For this review, take the finished solid that the model builds, in its own axes (mm). A direction names the side the tool comes from. Give positions to 0.01 mm unless a question says otherwise; leave off trailing zeros. Write each loop counter-clockwise with the first axis right and the second up, starting at its lowest first coordinate (ties: lowest second). Pieces come first, ordered by that corner, then holes.
1) We need section A-A on x = 13. Give the boundary of the cut face in (y, z), and give its area (3 significant figures).
2) Machinability: for faces 1 (the face through (24.53, 38.61, 4.93)), 2 (the face through (26.534, 92.543, 4.93)), which of the approach directions +Z, -Z, +X, -X, +Y, -Y give a long, thin tool a straight path to every point of the face, cutting with its end or side? Answer none if there is none.
3) We need section C-C on z = 5.5. Give the boundary of the cut face in (x, y).
4) We need section B-B on y = 65.5. Give the boundary of the cut face in (x, z).
5) Draft analysis for pull direction Y (two halves, no side actions). For faces 3 (the face through (26.525, 39.248, 4.93)), 4 (the face through (-49.662, 72.543, 4.93)), 5 (the face through (-52.564, 67, 5)), state which applies: pulls with the +Y half, pulls with the -Y half, needs draft (parallel to the pull), parting line crosses it, or undercut.
6) Wall thickness on line 1 along Y through (x, z) = (-12.5, 2); line 2 along X through (y, z) = (51, 7); line 3 along X through (y, z) = (73, 8.25): over which ranges is each line inside the solid? List them lowest first.
from build123d import *

# Parameters (mm, degrees)
RESSALTO_EXTRUS_O1_DEPTH = 10
CORTE_EXTRUS_O1_DEPTH    = 10


with BuildPart() as part:
    # Esboço1 → Ressalto-extrusão1 (new body)
    with BuildSketch(Plane.XY):
        with BuildLine():
            Line((-49.563885949, 93.398903013), (24.436114051, 93.398903013))
            ThreePointArc((24.436114051, 93.398903013), (26.557434395, 92.520223357), (27.436114051, 90.398903013))
            Line((27.436114051, 90.398903013), (27.436114051, 78.398903013))
            Line((27.436114051, 78.398903013), (27.436114051, 43.418903013))
            ThreePointArc((27.436114051, 43.418903013), (26.499191921, 39.192720396), (23.863990148, 35.758458582))
            Line((23.863990148, 35.758458582), (-48.991762046, 35.758458582))
            ThreePointArc((-48.991762046, 35.758458582), (-51.626963819, 39.192720396), (-52.563885949, 43.418903013))
            Line((-52.563885949, 43.418903013), (-52.563885949, 78.398903013))
            Line((-52.563885949, 78.398903013), (-52.563885949, 90.398903013))
            ThreePointArc((-52.563885949, 90.398903013), (-51.685206293, 92.520223357), (-49.563885949, 93.398903013))
        make_face()
    extrude(amount=RESSALTO_EXTRUS_O1_DEPTH)

    # Esboço2 → Corte-extrusão1 (cut)
    with BuildSketch(Plane(origin=(0, 0, 0), x_dir=(-1, 0, 0), z_dir=(0, 0, -1))):
        with BuildLine():
            Line((-22.436114051, 73.398903013), (47.563885949, 73.398903013))
            ThreePointArc((47.563885949, 73.398903013), (49.685206293, 72.520223357), (50.563885949, 70.398903013))
            Line((50.563885949, 70.398903013), (50.563885949, 40.758458582))
            ThreePointArc((50.563885949, 40.758458582), (49.685206293, 38.637138238), (47.563885949, 37.758458582))
            Line((47.563885949, 37.758458582), (-22.436114051, 37.758458582))
            ThreePointArc((-22.436114051, 37.758458582), (-24.557434395, 38.637138238), (-25.436114051, 40.758458582))
            Line((-25.436114051, 40.758458582), (-25.436114051, 70.398903013))
            ThreePointArc((-25.436114051, 70.398903013), (-24.557434395, 72.520223357), (-22.436114051, 73.398903013))
        make_face()
    extrude(amount=-CORTE_EXTRUS_O1_DEPTH, mode=Mode.SUBTRACT)


solid = part.part
Results list:
1. outline: (35.76, 0) - (37.76, 0) - (37.76, 10) - (35.76, 10) - close; (73.4, 0) - (93.4, 0) - (93.4, 10) - (73.4, 10) - close
1. area: 220 mm2
2. face 1: +Z, -Z
2. face 2: +Z, -Z, +X, +Y
3. outline: (-52.56, 43.42) arc R10 ccw to (-48.99, 35.76) - (23.86, 35.76) arc R10 ccw to (27.44, 43.42) - (27.44, 90.4) arc R3 ccw to (24.44, 93.4) - (-49.56, 93.4) arc R3 ccw to (-52.56, 90.4) - close; hole (-50.56, 40.76) arc R3 ccw to (-47.56, 37.76) - (22.44, 37.76) arc R3 ccw to (25.44, 40.76) - (25.44, 70.4) arc R3 ccw to (22.44, 73.4) - (-47.56, 73.4) arc R3 ccw to (-50.56, 70.4) - close
4. outline: (-52.56, 0) - (-50.56, 0) - (-50.56, 10) - (-52.56, 10) - close; (25.44, 0) - (27.44, 0) - (27.44, 10) - (25.44, 10) - close
5. face 3: pulls with the -Y half
5. face 4: undercut
5. face 5: needs draft
6. line 1: y = 35.76 to 37.76, 73.4 to 93.4
6. line 2: x = -52.56 to -50.56, 25.44 to 27.44
6. line 3: x = -52.56 to -49.06, 23.93 to 27.44
